Verification items for the finished model (mm, model axes). Face numbers are marked on the shaded views. Coordinates: 2 decimals unless noted, no trailing zeros. Loops run counter-clockwise (first coordinate to the right, second up) from the corner with the lowest first, then second, coordinate; pieces in that order, holes last. Notation, with made-up numbers: (32, -33) - (70, -33) arc R17 ccw to (70, -10) - close; hole circle Ø7 at (43, 54). An arc over 180 degrees is marked (long way). One line per item, written item: value. Start each with the question number.
(1) Draft check along X on the marked faces 1 and 2. Enter one of: +X half, -X half, draft (parallel to the pull), parting line (faces both ways), or undercut.
(2) Thickness scan on probe 1 along X at (y, z) = (5, -15); probe 2 along Z at (x, y) = (-20, 2); probe 3 along X at (y, z) = (0.7, -15). Record the ranges inside material, lowest first. Write a range as [from, to].
(3) Section check D-D (y = 0.5). Count the separate pieces of the cut face and the enclosed holes in it, plus the area to 3 significant figures.
(4) Section check C-C (x = -18). Record the boundary of the cut face in (y, z).
(5) Section check A-A (y = 5.75). Record the boundary of the cut face in (x, z), plus the area to 3 significant figures.
(6) Gauge pin test, flat ends, axial feed: P1, Ø3, axis at x = 1.59, z = -9.58, coming from the +Y side; P2, Ø4, axis at y = 2, z = 8, coming from the +X side; P3, Ø5, axis at x = -1, y = 2, coming from the +Z side; P4, Ø1.5, axis at x = 3, z = -0.5, coming from the +Y side. Record the tip position at first contact, or that the pin passes through.
(7) Section check B-B (z = 15). Record the boundary of the cut face in (x, y), plus the area to 3 significant figures.
```python
from build123d import *
from build123d.topology import SkipClean

# Parameters (mm, degrees)
SKETCH1_R               = 3
SKETCH1_R_2             = 1.7
BOSS_EXTRUDE1_DEPTH     = 10
BOSS_EXTRUDE1_2_DEPTH   = 10
BOSS_EXTRUDE1_3_DEPTH   = 10
BOSS_EXTRUDE1_4_DEPTH   = 10
BOSS_EXTRUDE2_DEPTH     = 2.5
CUT_EXTRUDE1_DEPTH      = 33.003906012
CUT_EXTRUDE1_DEPTH_BACK = 33.003906012
SKETCH1_2_R             = 1.7
SKETCH4_W               = 31.34314575
SKETCH4_H               = 20
BOSS_EXTRUDE3_DEPTH     = 2.5
FILLET2_R               = 1
BOSS_EXTRUDE4_DEPTH     = 2.5
CUT_EXTRUDE3_DEPTH      = 33.003906012
CUT_EXTRUDE3_DEPTH_BACK = 33.003906012
SKETCH5_R               = 1.55
FILLET3_R               = 3


with BuildPart() as part:
    # Sketch1 → Boss-Extrude1 (new body)
    with BuildSketch(Plane(origin=(0, 0, 0), x_dir=(1, 0, 0), z_dir=(0, 1, 0))):
        with Locations(Location((-21.5, 15, 0), (0, 0, 270))):
            Circle(SKETCH1_R)
        with Locations(Location((-21.5, 15, 0), (0, 0, 270))):
            Circle(SKETCH1_R_2, mode=Mode.SUBTRACT)
    extrude(amount=BOSS_EXTRUDE1_DEPTH)



with BuildPart() as body_2:
    # Sketch1 → Boss-Extrude1 2 (new body)
    with BuildSketch(Plane(origin=(0, 0, 0), x_dir=(1, 0, 0), z_dir=(0, 1, 0))):
        with Locations(Location((-21.5, -15, 0), (0, 0, 270))):
            Circle(SKETCH1_R)
        with Locations(Location((-21.5, -15, 0), (0, 0, 270))):
            Circle(SKETCH1_R_2, mode=Mode.SUBTRACT)
    extrude(amount=BOSS_EXTRUDE1_2_DEPTH)


with BuildPart() as body_3:
    # Sketch1 → Boss-Extrude1 3 (new body)
    with BuildSketch(Plane(origin=(0, 0, 0), x_dir=(1, 0, 0), z_dir=(0, 1, 0))):
        with Locations(Location((21.5, -15, 0), (0, 0, 270))):
            Circle(SKETCH1_R)
        with Locations(Location((21.5, -15, 0), (0, 0, 270))):
            Circle(SKETCH1_R_2, mode=Mode.SUBTRACT)
    extrude(amount=BOSS_EXTRUDE1_3_DEPTH)


with BuildPart() as body_4:
    # Sketch1 → Boss-Extrude1 4 (new body)
    with BuildSketch(Plane(origin=(0, 0, 0), x_dir=(1, 0, 0), z_dir=(0, 1, 0))):
        with Locations(Location((21.5, 15, 0), (0, 0, 270))):
            Circle(SKETCH1_R)
        with Locations(Location((21.5, 15, 0), (0, 0, 270))):
            Circle(SKETCH1_R_2, mode=Mode.SUBTRACT)
    extrude(amount=BOSS_EXTRUDE1_4_DEPTH)


with BuildPart() as part_1:
    with SkipClean():  # the faces are left unmerged after this step: merging them gives an invalid solid
        add(part.part)

        add(body_2.part)  # Boss-Extrude2 merges body 2

        add(body_3.part)  # Boss-Extrude2 merges body 3

        add(body_4.part)  # Boss-Extrude2 merges body 4
        # Sketch2 → Boss-Extrude2 (add)
        with BuildSketch(Plane(origin=(0, 0, 0), x_dir=(1, 0, 0), z_dir=(0, 1, 0))):
            with BuildLine():
                Line((-15.671572875, 12.171572875), (-15.671572875, -12.171572875))
                ThreePointArc((-15.671572875, -12.171572875), (-15.899934278, -13.319623172), (-16.550252532, -14.292893219))
                Line((-16.550252532, -14.292893219), (-19.378679656, -17.121320344))
                ThreePointArc((-19.378679656, -17.121320344), (-23.621320344, -17.121320344), (-23.621320344, -12.878679656))
                Line((-23.621320344, -12.878679656), (-21.671572875, -10.928932188))
                Line((-21.671572875, -10.928932188), (-21.671572875, 10.928932188))
                Line((-21.671572875, 10.928932188), (-23.621320344, 12.878679656))
                ThreePointArc((-23.621320344, 12.878679656), (-23.621320344, 17.121320344), (-19.378679656, 17.121320344))
                Line((-19.378679656, 17.121320344), (-16.550252532, 14.292893219))
                ThreePointArc((-16.550252532, 14.292893219), (-15.899934278, 13.319623172), (-15.671572875, 12.171572875))
            make_face()
            with BuildLine():
                ThreePointArc((19.378679656, 17.121320344), (23.621320344, 17.121320344), (23.621320344, 12.878679656))
                Line((23.621320344, 12.878679656), (21.671572875, 10.928932188))
                Line((21.671572875, 10.928932188), (21.671572875, -10.928932188))
                Line((21.671572875, -10.928932188), (23.621320344, -12.878679656))
                ThreePointArc((23.621320344, -12.878679656), (23.621320344, -17.121320344), (19.378679656, -17.121320344))
                Line((19.378679656, -17.121320344), (16.550252532, -14.292893219))
                ThreePointArc((16.550252532, -14.292893219), (15.899934278, -13.319623172), (15.671572875, -12.171572875))
                Line((15.671572875, -12.171572875), (15.671572875, 12.171572875))
                ThreePointArc((15.671572875, 12.171572875), (15.899934278, 13.319623172), (16.550252532, 14.292893219))
                Line((16.550252532, 14.292893219), (19.378679656, 17.121320344))
            make_face()
        extrude(amount=BOSS_EXTRUDE2_DEPTH)

    # Sketch1<2> → Cut-Extrude1 (cut, two sides: drawn at the far end of the back side and taken through both)
    with SkipClean():  # the faces are left unmerged after this step: merging them gives an invalid solid
        with BuildSketch(Plane(origin=(0, 0, 0), x_dir=(1, 0, 0), z_dir=(0, 1, 0)).offset(-CUT_EXTRUDE1_DEPTH_BACK)):
            with Locations(Location((-21.5, -15, 0), (0, 0, 270))):
                Circle(SKETCH1_2_R)
            with Locations(Location((-21.5, 15, 0), (0, 0, 270))):
                Circle(SKETCH1_2_R)
            with Locations(Location((21.5, 15, 0), (0, 0, 270))):
                Circle(SKETCH1_2_R)
            with Locations(Location((21.5, -15, 0), (0, 0, 270))):
                Circle(SKETCH1_2_R)
        extrude(amount=CUT_EXTRUDE1_DEPTH + CUT_EXTRUDE1_DEPTH_BACK, mode=Mode.SUBTRACT)

    # Sketch4 → Boss-Extrude3 (add)
    with SkipClean():  # the faces are left unmerged after this step: merging them gives an invalid solid
        with BuildSketch(Plane(origin=(0, 0, 0), x_dir=(1, 0, 0), z_dir=(0, 1, 0))):
            Rectangle(SKETCH4_W, SKETCH4_H)
        extrude(amount=BOSS_EXTRUDE3_DEPTH)

    # Fillet2
    fillet2_edges = [part_1.edges().sort_by_distance(p)[0] for p in [
        (15.671572875, 1.25, 10),
        (15.671572875, 1.25, -10),
        (-15.671572875, 1.25, -10),
        (-15.671572875, 1.25, 10),
    ]]
    fillet(fillet2_edges, radius=FILLET2_R)

    # Sketch6 → Boss-Extrude4 (add)
    with SkipClean():  # the faces are left unmerged after this step: merging them gives an invalid solid
        with BuildSketch(Plane.XZ):
            Polygon((1.590990258, -4.16259377), (-3.827712857, -9.581296885), (1.590990258, -15), (7.009693373, -9.581296885), align=None)
            Polygon((-1.590990258, 15), (-9.445268772, 7.145721485), (-1.590990258, -0.70855703), (6.263288257, 7.145721485), align=None)
        extrude(amount=-BOSS_EXTRUDE4_DEPTH)

    # Sketch5 → Cut-Extrude3 (cut, two sides: drawn at the far end of the back side and taken through both)
    with SkipClean():  # the faces are left unmerged after this step: merging them gives an invalid solid
        with BuildSketch(Plane.XZ.offset(-CUT_EXTRUDE3_DEPTH_BACK)):
            with Locations(Location((-9.581296885, 1.590990258, 0), (0, 0, 90))):
                Circle(SKETCH5_R)
            with Locations(Location((1.590990258, -9.581296885, 0), (0, 0, 90))):
                Circle(SKETCH5_R)
            with BuildLine():
                Line((-0.671751442, 10.641957057), (10.641957057, -0.671751442))
                ThreePointArc((10.641957057, -0.671751442), (10.641957057, -2.793071786), (8.520636713, -2.793071786))
                Line((8.520636713, -2.793071786), (-2.793071786, 8.520636713))
                ThreePointArc((-2.793071786, 8.520636713), (-2.793071786, 10.641957057), (-0.671751442, 10.641957057))
            make_face()
        extrude(amount=CUT_EXTRUDE3_DEPTH + CUT_EXTRUDE3_DEPTH_BACK, mode=Mode.SUBTRACT)

    # Fillet3
    fillet3_edges = [part_1.edges().sort_by_distance(p)[0] for p in [
        (1.590990258, 1.25, -15),
        (-1.590990258, 1.25, 15),
    ]]
    fillet(fillet3_edges, radius=FILLET3_R)


solid = part_1.part
```
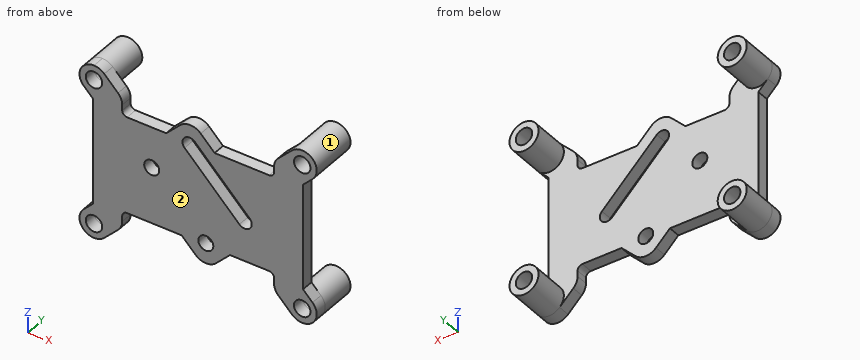
Responses:
1. face 1: undercut
1. face 2: draft
2. probe 1: x = [-24.5, -23.2], [-19.8, -18.5], [18.5, 19.8], [23.2, 24.5]
2. probe 2: z = [-17.6, -15.8], [-14.2, 14.2], [15.8, 17.6]
2. probe 3: x = [-24.5, -23.2], [-19.8, -17.26], [17.26, 19.8], [23.2, 24.5]
3. separate pieces: 1
3. enclosed holes: 7
3. area: 1,010 mm²
4. outline: (0, -15.74) - (2.5, -15.74) - (2.5, 15.74) - (0, 15.74) - close
5. outline: circle Ø6 at (-21.5, -15); circle Ø6 at (-21.5, 15); circle Ø6 at (21.5, -15); circle Ø6 at (21.5, 15); hole circle Ø3.4 at (-21.5, -15); hole circle Ø3.4 at (-21.5, 15); hole circle Ø3.4 at (21.5, -15); hole circle Ø3.4 at (21.5, 15)
5. area: 76.8 mm²
6. P1: passes through
6. P2: stops at x = 21.67
6. P3: stops at z = 13.76
6. P4: stops at y = 2.5
7. outline: (-24.5, 0) - (-23.2, 0) - (-23.2, 10) - (-24.5, 10) - close; (-19.8, 0) - (-17.26, 0) - (-17.26, 2.5) - (-18.5, 2.5) - (-18.5, 10) - (-19.8, 10) - close; (17.26, 0) - (19.8, 0) - (19.8, 10) - (18.5, 10) - (18.5, 2.5) - (17.26, 2.5) - close; (23.2, 0) - (24.5, 0) - (24.5, 10) - (23.2, 10) - close
7. area: 58.2 mm²
